Input: part model. Units: mm. Frame: model coordinates. A direction names the side the tool comes from. Give positions to 0.01 mm unless a question says otherwise; leave off trailing zeros. Loops run counter-clockwise (first coordinate to the right, second up) from the corner with the lowest first, then second, coordinate; pieces in that order, holes last. Notation, with made-up numbers: M 88.5,82.25 L 92.5,82.25 A20 ccw 92.5,106.25 Z; hole C 45.25,-14.75 d10. An arc over 180 degrees is marked long. Return JSON: item names as keys, results as strings. Group by question number.
```python
from build123d import *

# Parameters (mm, degrees)
F1_DEPTH       = 460
F3_D           = 5.5
F3_CBORE_D     = 9.75
F3_CBORE_DEPTH = 5


with BuildPart() as f1:
    # F0 (on Front) → F1 (new body)
    with BuildSketch(Plane.XZ):
        with BuildLine():
            Line((-7.5, 2.1513768696), (-7.5, 0))
            Line((-7.5, 0), (7.5, 0))
            Line((7.5, 0), (7.5, 2.1513768696))
            ThreePointArc((7.5, 2.1513768696), (4.59, 6), (7.5, 9.8486231304))
            Line((7.5, 9.8486231304), (7.5, 11.2))
            Line((7.5, 11.2), (5.5, 13.2))
            Line((5.5, 13.2), (-5.5, 13.2))
            Line((-5.5, 13.2), (-7.5, 11.2))
            Line((-7.5, 11.2), (-7.5, 9.8486231304))
            ThreePointArc((-7.5, 9.8486231304), (-4.59, 6), (-7.5, 2.1513768696))
        make_face()
    extrude(amount=F1_DEPTH)

    # F3 (through all)
    with Locations(Plane.XY.offset(13.2)):
        with Locations((0, -20), (0, -80), (0, -140), (0, -200), (0, -260), (0, -320), (0, -380), (0, -440)):
            CounterBoreHole(F3_D / 2, F3_CBORE_D / 2, F3_CBORE_DEPTH)


solid = f1.part
```
Item 1: First-contact query: pin 1 Ø4.5 at (x, y) = (0, -380) entering from -Z; pin 2 Ø5 at (x, y) = (-0.5, -20) entering from +Z; pin 3 Ø2 at (y, z) = (-393, 6.5) entering from -X. Flat tips, straight axial feed; report the tip coordinate or a pass-through.
Item 2: Pull-direction query (Y, two-part tool) for faces 1 (the face through (0, 0, 7)), 2 (the face through (0, -227, 13.2)), 3 (the face through (-1.06, -384.76, 10.74)); classes: pulls with the +Y half, pulls with the -Y half, needs draft (parallel to the pull), parting line crosses it, or undercut.
Item 3: Reachability of faces 4 (the face through (-0.635, -195.166, 10.735)), 5 (the face through (0, -227, 0)) from +Z, -Z, +X, -X, +Y, -Y: full face, straight path, thin tool, end or side. Return the list, or none.
Item 4: Section B-B, the plane y = -223. Return loops of the section in (x, z).
Item 5: Section A-A, the plane z = 6. Give the number of separate pieces and of enclosed holes in the cut face, then the cut area to 3 significant figures.
Item 6: Material intervals for line 1 (X direction, y = -320, z = 6); line 2 (Z direction, x = -6, y = -72); line 3 (X direction, y = -42, z = 6.5), sorted ascending. Write a range as from..to.
Answer below:
{
 "1": {"pin 1": "through", "pin 2": "z = 8.2", "pin 3": "x = -4.88"},
 "2": {"face 1": "pulls with the +Y half", "face 2": "needs draft", "face 3": "undercut"},
 "3": {"face 4": "+Z", "face 5": "-Z, +X, -X, +Y, -Y"},
 "4": {"outline": "M -7.5,0 L 7.5,0 L 7.5,2.15 A4 cw 7.5,9.85 L 7.5,11.2 L 5.5,13.2 L -5.5,13.2 L -7.5,11.2 L -7.5,9.85 A4 cw -7.5,2.15 Z"},
 "5": {"separate pieces": "1", "enclosed holes": "8", "area": "4,030 mm^2"},
 "6": {"line 1": "-4.59..-2.75, 2.75..4.59", "line 2": "0..2.95, 9.05..12.7", "line 3": "-4.62..4.62"}
}
